Autodesk Inventor part; units mm, degrees
ref_plane "YZ Plane" through (0, 0, 0) normal (1, 0, 0) x (0, 1, 0)
ref_plane "XZ Plane" through (0, 0, 0) normal (0, 1, 0) x (-1, 0, 0)
ref_plane "XY Plane" through (0, 0, 0) normal (0, 0, 1) x (1, 0, 0)
sketch "Sketch1" plane through (0, 0, 0) normal (0, 0, 1) x (1, 0, 0)
  line L0 (12, 0) -> (-12, 0)
  line L1 (-12, 0) -> (-12, 1.6)
  line L2 (-12, 1.6) -> (4, 9.6)
  line L3 (4, 9.6) -> (12, 9.6)
  line L4 (12, 9.6) -> (12, 0)
  point P0 (0, 0)
  point P1 (0, 0)
  dimension "d0" = 9.6
  dimension "d1" = 24
  dimension "d2" = 16
  dimension "d3" = 1.6
extrude "Extrusion1" add sketch "Sketch1" along normal mid plane 16
shell "Shell1" thickness 0.8 removed faces 1 at (-4, 0, 2.6667)
sketch "Sketch2" plane through (4, 9.6, 8) normal (0, 1, 0) x (1, 0, 0)
  line L0 (4, 12) -> (4, 4) construction
  line L1 (-20.8, 8) -> (12.8, 8) construction
  line L2 (8, 0) -> (8, 16) construction
  circle A0 centre (4, 12) radius 2.5
  circle A1 centre (4, 4) radius 2.5
  point P0 (4, 8)
  dimension "d6" = 4
  dimension "d7" = 8
  dimension "d8" = 5
extrude "Extrusion2" add sketch "Sketch2" along normal blind 1.6
properties part number "LEGO Brick 3298" material "Steel"
Can you work these out from the model? Positions are in its coordinate system, mm. A direction names the side the tool comes from. Give positions to 0.01 mm unless a question says otherwise; leave off trailing zeros. Order: outer loops, then holes, each group sorted by start corner. A loop starts at its lowest first (then second) coordinate and runs counter-clockwise, first axis right, second up. Notation, with made-up numbers: M -29,-9.5 L 15,-9.5 A24 cw 15,15.5 Z; hole C -26.75,59 d5. An arc over 180 degrees is marked long. Write item = value, one per line. Start each with the question number.
Q1. Suppose I cut it at A-A (z = -4). Write out the boundary of the cut face in (x, y), plus the area to 3 significant figures.
Q2. Suppose I cut it at C-C (x = 2). Write out the boundary of the cut face in (y, z).
Q3. I need wall thicknesses on probe 1 along Z at (x, y) = (-0.75, 5.5); probe 2 along X at (y, z) = (0.75, -6); probe 3 along Y at (x, z) = (8.5, 6). Which ranges of each line are inside material? Lowest first, please. Write a range as [from, to].
Q4. Will these pins go through, and if not, where does the flat tip stop? pin 1 Ø5.5 at (x, z) = (6.5, 1.5) entering from -Y; pin 2 Ø1 at (x, y) = (-5, 6) entering from -Z; pin 3 Ø3 at (y, z) = (8, -0.5) entering from -X; pin 4 Ø5 at (x, z) = (7.5, -6) entering from -Y.
Q5. For faces 5 (the flat face through (2, 4, -8)), 6 (the cylindrical face through (10.385, 10.389, 4.751)), 7 (the flat face through (-3.61, 4.9, -0.1)), which set-ups out of +Z, -Z, +X, -X, +Y, -Y let a thin tool reach every point of the face, with its end or its side?
Q6. Suppose I cut it at D-D (z = 0.25). Write out the boundary of the cut face in (x, y).
Q7. We'd pull the mould along Z, two halves only. Please class faces 1 (the flat face through (2, 4, 8)), 2 (the flat face through (2, 3, -7.2)), 3 (the flat face through (11.2, 4, 0)), 4 (the flat face through (-4.112, 5.544, -0.112)): pulls with the +Z half, pulls with the -Z half, needs draft (parallel to the pull), parting line crosses it, or undercut.
Q8. Suppose I cut it at B-B (y = 4). Write out the boundary of the cut face in (x, z).
Check result:
q1.outline = M -12,0 L -11.2,0 L -11.2,1.11 L 4.19,8.8 L 11.2,8.8 L 11.2,0 L 12,0 L 12,9.6 L 10.5,9.6 L 10.5,11.2 L 5.5,11.2 L 5.5,9.6 L 4,9.6 L -12,1.6 Z
q1.area = 36.5 mm2
q2.outline = M 0,-8 L 8.6,-8 L 8.6,8 L 0,8 L 0,7.2 L 7.71,7.2 L 7.71,-7.2 L 0,-7.2 Z
q3.probe_1 = [-8, -7.2], [7.2, 8]
q3.probe_2 = [-12, -11.2], [11.2, 12]
q3.probe_3 = [8.8, 11.2]
q4.pin_1 = 8.58
q4.pin_2 = through
q4.pin_3 = -2.2
q4.pin_4 = 0
q5.face_5 = -Z, +X, -X, +Y, -Y
q5.face_6 = +Y
q5.face_7 = -Y
q6.outline = M -12,0 L -11.2,0 L -11.2,1.11 L 4.19,8.8 L 11.2,8.8 L 11.2,0 L 12,0 L 12,9.6 L 4,9.6 L -12,1.6 Z
q7.face_1 = pulls with the +Z half
q7.face_2 = undercut
q7.face_3 = undercut
q7.face_4 = needs draft
q8.outline = M -7.2,-8 L 12,-8 L 12,8 L -7.2,8 Z; hole M -5.41,-7.2 L 11.2,-7.2 L 11.2,7.2 L -5.41,7.2 Z
